Part print with two shaded views. Sizes in mm from the minimum x, y, z corner. Round coordinates to 2 decimals unless told otherwise and drop trailing zeros. Write each loop counter-clockwise with the first axis right and the second up, starting at its lowest first coordinate (ties: lowest second). Pieces come first, ordered by that corner, then holes. Notation, with made-up numbers: (73, 35) -> (116, 35) arc R12 cw to (116, 43) -> close; hole circle Ø11 at (52.25, 8). An arc over 180 degrees is marked (long way). Answer as CSV lines item,"result".
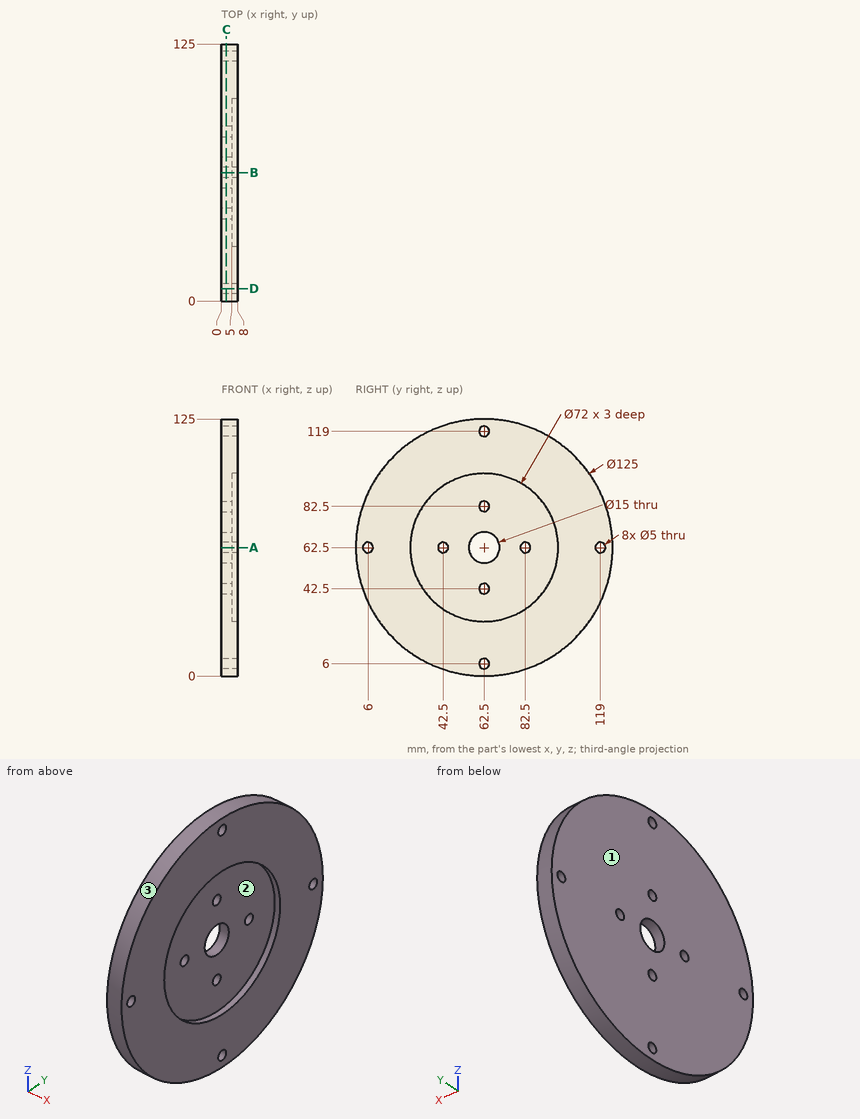
1. Cut at A-A, the plane z = 62.5. Write the cut outline in (x, y), then the cut area to 3 significant figures.
Results found:
outline,"(0, 0) -> (8, 0) -> (8, 3.5) -> (0, 3.5) -> close; (0, 8.5) -> (8, 8.5) -> (8, 26.5) -> (5, 26.5) -> (5, 40) -> (0, 40) -> close; (0, 45) -> (5, 45) -> (5, 55) -> (0, 55) -> close; (0, 70) -> (5, 70) -> (5, 80) -> (0, 80) -> close; (0, 85) -> (5, 85) -> (5, 98.5) -> (8, 98.5) -> (8, 116.5) -> (0, 116.5) -> close; (0, 121.5) -> (8, 121.5) -> (8, 125) -> (0, 125) -> close"
area,"579 mm2"
2. Cut at D-D, the plane y = 6. Write the cut outline in (x, z), then the cut area to 3 significant figures.
Results found:
outline,"(0, 35.78) -> (8, 35.78) -> (8, 60) -> (0, 60) -> close; (0, 65) -> (8, 65) -> (8, 89.22) -> (0, 89.22) -> close"
area,"388 mm2"
3. Drop flat-ended pins along their axis: pin 1 Ø21.5 at (y, z) = (70.5, 45) entering from +X; pin 2 Ø4 at (x, y) = (5.5, 84.5) entering from -Z; pin 3 Ø4 at (x, z) = (1, 85.5) entering from +Y. Give the stop position or say it passes through.
Results found:
pin 1,"stops at x = 5"
pin 2,"stops at z = 3.29"
pin 3,"stops at y = 121.37"
4. Probe line 1 along Z through (x, y) = (3.15, 62.5); line 2 along Z through (x, y) = (7, 62.5); line 3 along X through (y, z) = (58, 36.5). List the from-to ranges inside material, lowest first.
Results found:
line 1,"z = 0 to 3.5, 8.5 to 40, 45 to 55, 70 to 80, 85 to 116.5, 121.5 to 125"
line 2,"z = 0 to 3.5, 8.5 to 26.5, 98.5 to 116.5, 121.5 to 125"
line 3,"x = 0 to 5"
5. Mould opens along Z. For the marked faces 1, 2 and 3 say: +Z half, -Z half, draft (parallel to the pull), parting line (faces both ways), or undercut.
Results found:
face 1,"draft"
face 2,"undercut"
face 3,"parting line"
6. Cut at C-C, the plane x = 2.5. Count the separate pieces of the cut face and the enclosed holes in it, then the cut area to 3 significant figures.
Results found:
separate pieces,"1"
enclosed holes,"9"
area,"11,900 mm2"
